from build123d import *

# Parameters (mm, degrees)
F0_R     = 37.5
F0_R_2   = 10
F1_DEPTH = 10
F3_DEPTH = 10
F4_W     = 54.9519052838
F4_H     = 2.5
F5_DEPTH = 300
F6_DEPTH = 20


with BuildPart() as f1:
    # F0 (on Top) → F1 (new body)
    with BuildSketch(Plane.XY):
        with Locations((-117.0892864466, -13.0537990481)):
            Circle(F0_R)
        with Locations((-117.0892864466, -13.0537990481)):
            Circle(F0_R_2, mode=Mode.SUBTRACT)
        with Locations((-117.0892864466, -13.0537990481)):
            Circle(F0_R_2)
    extrude(amount=F1_DEPTH)

    # F2 (on face) → F3 (join)
    with BuildSketch(Plane.XY.offset(10)):
        Polygon((-144.0126514019, -39.1571018943), (-81.0214805814, -23.3184656317), (-126.2337273564, 23.3141703817), align=None)
    extrude(amount=F3_DEPTH)

    # F4 (on face) → F5 (join)
    with BuildSketch(Plane(origin=(0.6967599266, -2.7710544537, 0), x_dir=(0.9698125181, 0.2438517576, 0), z_dir=(0.2438517576, -0.9698125181, 0))):
        with Locations((-116.7378475757, 16.25)):
            Rectangle(F4_W, F4_H)
    extrude(amount=F5_DEPTH)

    # F0 (on Top) → F6 (join)
    with BuildSketch(Plane.XY):
        with Locations((-117.0892864466, -13.0537990481)):
            Circle(F0_R_2)
    extrude(amount=-F6_DEPTH)


solid = f1.part
Could you check a few things on this model? Use its own coordinates, in mm. A direction names the side the tool comes from. Round coordinates to 2 decimals unless told otherwise and drop trailing zeros. Write each loop counter-clockwise with the first axis right and the second up, starting at its lowest first coordinate (ties: lowest second). Pieces come first, ordered by that corner, then holes. Notation, with made-up numbers: (28, 19) - (36, 19) arc R15 cw to (36, 43) - close; hole circle Ø5 at (87.25, -9.75). An arc over 180 degrees is marked (long way). Put each result on its own line as item: value. Start each with the question number.
(1) I want a section at B-B, the plane x = -43.5. Please give me the cut outline in (y, z), plus the area to 3 significant figures.
(2) I want a section at A-A, the plane y = -29. Please give me the cut outline in (x, z), plus the area to 3 significant figures.
(3) I want a section at D-D, the plane x = -62. Please give me the cut outline in (y, z).
(4) I need wall thicknesses on probe 1 along Z at (x, y) = (-55, -203.5); probe 2 along Z at (x, y) = (-97, -25); probe 3 along Y at (x, z) = (-109, 3). Which ranges of each line are inside material? Lowest first, please.
(5) For faces 4 (the flat face through (-134.999, -7.484, 14.93)), 5 (the cylindrical face through (-107.85, -16.88, -9.86)), 6 (the flat face through (-103.31, -0.33, 14.93)), 7 (the flat face through (-113, -40, 10)), 8 (the flat face through (-117, -13, -20)), which set-ups out of +Z, -Z, +X, -X, +Y, -Y let a thin tool reach every point of the face, with its end or its side?
(6) Will these pins go through, and if not, where does the flat tip stop? pin 1 (4 mm diameter, centred on x = -136.5, z = 1.5, fed in from +Y); pin 2 (3 mm diameter, centred on x = -83.5, y = -196.5, fed in from +Z); pin 3 (5 mm diameter, centred on x = -39.5, y = -241, fed in from -Z); pin 4 (10 mm diameter, centred on y = -67.5, z = 6.5, fed in from +X).
(7) Thinking about a two-plate mould opening in Z: for faces 1 (the flat face through (-39.735, -322.275, 16.267)), 2 (the flat face through (-112.96, -31.35, 13.82)), 3 (the flat face through (-120, -14, 20)), which applies, released by +Z, released by -Z, zero draft, split by the parting line, or undercut?
(8) I want a section at C-C, the plane z = -3.5. Please give me the cut outline in (x, y), plus the area to 3 significant figures.
Here are the results:
1. outline: (-323.22, 15) - (-193.05, 15) - (-193.05, 17.5) - (-323.22, 17.5) - close
1. area: 325 mm^2
2. outline: (-151.03, 0) - (-83.15, 0) - (-83.15, 10) - (-103.62, 10) - (-103.62, 15) - (-84.75, 15) - (-84.75, 17.5) - (-103.62, 17.5) - (-103.62, 20) - (-141.12, 20) - (-141.12, 10) - (-151.03, 10) - close
2. area: 1,100 mm^2
3. outline: (-327.87, 15) - (-119.47, 15) - (-119.47, 17.5) - (-327.87, 17.5) - close
4. probe 1: z = 15 to 17.5
4. probe 2: z = 0 to 20
4. probe 3: y = -49.67 to 23.56
5. face 4: +Z, -X, +Y
5. face 5: -Z
5. face 6: +Z, +X, +Y
5. face 7: +X, -Y
5. face 8: -Z, +X, -X, +Y, -Y
6. pin 1: stops at y = 20.16
6. pin 2: stops at z = 17.5
6. pin 3: stops at z = 15
6. pin 4: passes through
7. face 1: zero draft
7. face 2: undercut
7. face 3: released by +Z
8. outline: circle Ø20 at (-117.09, -13.05)
8. area: 314 mm^2
